Geometry check sheet. Reference: drawing and pictorial views, mm from the part's lowest x, y, z. A direction names the side the tool comes from. Round coordinates to 2 decimals unless told otherwise and drop trailing zeros. Write each loop counter-clockwise with the first axis right and the second up, starting at its lowest first coordinate (ties: lowest second). Pieces come first, ordered by that corner, then holes. Notation, with made-up numbers: M -25.75,3.25 L 4.25,3.25 A16 cw 4.25,22.25 Z; hole C -8,-23.5 d8. An arc over 180 degrees is marked long. Answer in a Markdown table with one row per item.
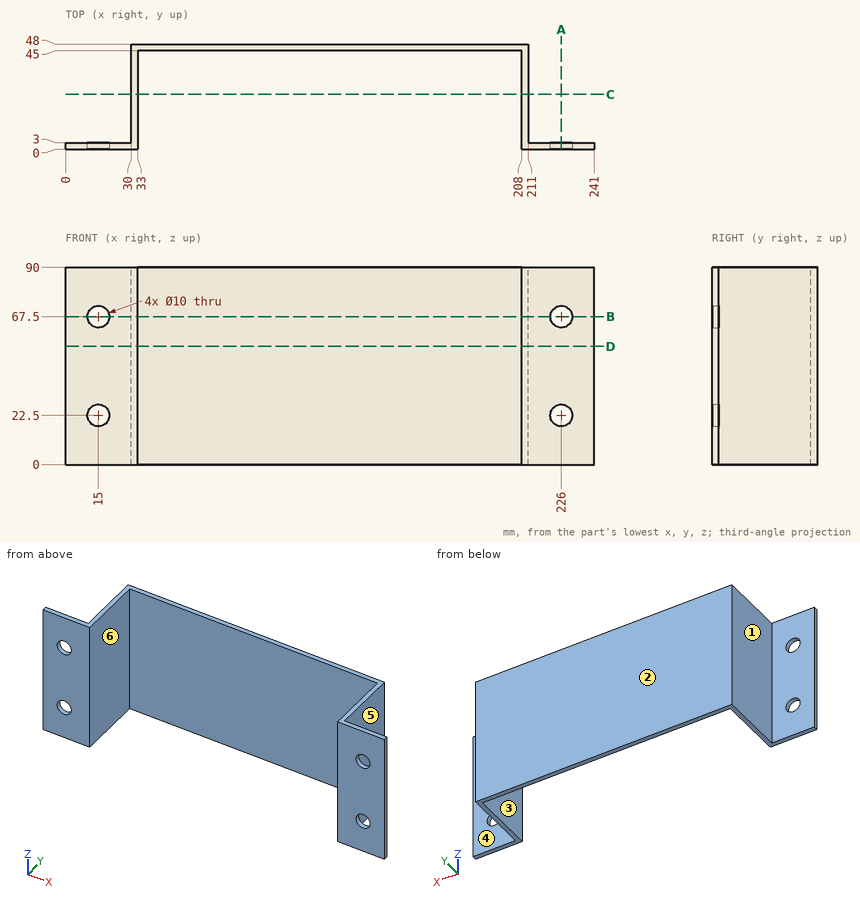
1. Access from +Z, -Z, +X, -X, +Y, -Y to the whole of each face (thin tool, end or side, straight path). Record for the marked faces 1, 2 and 3.
Found:
| item | result |
|---|---|
| face 1 | +Z, -Z, -X, +Y |
| face 2 | +Z, -Z, +X, -X, +Y |
| face 3 | +Z, -Z, -Y |
2. Section check C-C, the plane y = 25. Record the cut outline in (x, z), and give its area (3 significant figures).
Found:
| item | result |
|---|---|
| outline | M 30,0 L 33,0 L 33,90 L 30,90 Z; M 208,0 L 211,0 L 211,90 L 208,90 Z |
| area | 540 mm2 |
3. Draft check along X on the marked faces 4, 5 and 6. Enter one of: +X half, -X half, draft (parallel to the pull), parting line (faces both ways), or undercut.
Found:
| item | result |
|---|---|
| face 4 | draft |
| face 5 | +X half |
| face 6 | undercut |
4. Section check D-D, the plane z = 54. Record the cut outline in (x, y), and give its area (3 significant figures).
Found:
| item | result |
|---|---|
| outline | M 0,0 L 33,0 L 33,45 L 208,45 L 208,0 L 241,0 L 241,3 L 211,3 L 211,48 L 30,48 L 30,3 L 0,3 Z |
| area | 993 mm2 |
5. Go/stop test with flat-tipped pins: pin 1 (9 mm diameter, centred on x = 15, z = 67.5, fed in from -Y); pin 2 (11.5 mm diameter, centred on x = 15, z = 22.5, fed in from -Y); pin 3 (24 mm diameter, centred on x = 15.5, z = 50.5, fed in from +Y); pin 4 (13.5 mm diameter, centred on y = 26, z = 63, fed in from -X). Record where each tip stops, or that it passes through.
Found:
| item | result |
|---|---|
| pin 1 | passes through |
| pin 2 | stops at y = 0 |
| pin 3 | stops at y = 3 |
| pin 4 | stops at x = 30 |
6. Scan lines: L1, parallel to X at y = 1.25, z = 22.5; L2, parallel to Z at x = 15, y = 1.1; L3, parallel to X at y = 10, z = 14.5. Record each from-to range of solid material in increasing order.
Found:
| item | result |
|---|---|
| L1 | x = 0 to 10, 20 to 33, 208 to 221, 231 to 241 |
| L2 | z = 0 to 17.5, 27.5 to 62.5, 72.5 to 90 |
| L3 | x = 30 to 33, 208 to 211 |
7. Section check B-B, the plane z = 67.5. Record the cut outline in (x, y), and give its area (3 significant figures).
Found:
| item | result |
|---|---|
| outline | M 0,0 L 10,0 L 10,3 L 0,3 Z; M 20,0 L 33,0 L 33,45 L 208,45 L 208,0 L 221,0 L 221,3 L 211,3 L 211,48 L 30,48 L 30,3 L 20,3 Z; M 231,0 L 241,0 L 241,3 L 231,3 Z |
| area | 933 mm2 |
8. Section check A-A, the plane x = 226. Record the cut outline in (y, z), and give its area (3 significant figures).
Found:
| item | result |
|---|---|
| outline | M 0,0 L 3,0 L 3,17.5 L 0,17.5 Z; M 0,27.5 L 3,27.5 L 3,62.5 L 0,62.5 Z; M 0,72.5 L 3,72.5 L 3,90 L 0,90 Z |
| area | 210 mm2 |
